Here's how the part is built. I have some questions about the finished solid (model axes, mm). A direction names the side the tool comes from. Coordinates: 2 decimals unless noted, no trailing zeros. Write each loop counter-clockwise with the first axis right and the second up, starting at its lowest first coordinate (ties: lowest second). Pieces come first, ordered by that corner, then holes.
Item 1: I want a section at A-A (y = 8.75). Please give me the cut outline in (x, z).
Item 2: I want a section at B-B (y = 13). Please give me the cut outline in (x, z), and give its area (3 significant figures).
Item 3: I'm going to push flat-ended pins straight in: P1, Ø2, axis at y = 12.5, z = 1.5, coming from the -X side; P2, Ø1, axis at x = 4, y = 5, coming from the -Z side; P3, Ø3, axis at x = -11.5, y = 6, coming from the +Z side. Where does each tip first touch, or does it pass through?
Item 4: Please list where these lines run through material, in increasing order: line 1 (Y direction, x = 16.5, z = 5); line 2 (Y direction, x = 9, z = 14); line 3 (Y direction, x = -8.5, z = 13).
Item 5: For faces 1 (the face through (-12.65, 4.54, -8.06)), 2 (the face through (5.4, 16.5, 16.4)), 3 (the face through (5.4, 5, -16.4)), which set-ups out of +Z, -Z, +X, -X, +Y, -Y let a thin tool reach every point of the face, with its end or its side?
Item 6: If we mould it in two halves opening along X, with no side actions, what happens to faces 4 (the face through (12.4, 1, -6.5)), 5 (the face through (11, 8, -11)), 6 (the face through (11, 0, -9)), 7 (the face through (16.41, 2.23, -8.54))? For each: pulls with the +X half, pulls with the -X half, needs draft (parallel to the pull), parting line crosses it, or undercut.
from build123d import *

# Parameters (mm, degrees)
CHAMFER_1_SIZE = 0.5


with BuildPart() as part:
    # 草图1 → 旋转1 (revolve)
    with BuildSketch(Plane.XY, mode=Mode.PRIVATE) as revolve_1_sk:
        Polygon((14, 0), (14, 2), (15, 2), (15, 7), (16.15, 7), (16.15, 8), (15, 8), (15, 11), (17.65, 11), (17.65, 12), (16.5, 12), (16.5, 16.5), (18.55, 16.5), (19.05, 16), (19.05, 5.5), (18.55, 5), (17, 5), (17, 4), (18.5, 4), (18.5, 0.5), (18, 0), align=None)
    revolve(revolve_1_sk.sketch.rotate(Axis((0, 0, 0), (0, 1, 0)), 90), axis=Axis((0, 0, 0), (0, 1, 0)))  # turned: the seam where the file's is

    # 倒角1
    chamfer_1_edges = [part.edges().sort_by_distance(p)[0] for p in [
        (0, 11, 15),
        (0, 16.5, 16.5),
    ]]
    chamfer(chamfer_1_edges, length=CHAMFER_1_SIZE)


solid = part.part
Answer:
1. outline: circle Ø38.1 at (0, 0); hole circle Ø30 at (0, 0)
2. outline: circle Ø38.1 at (0, 0); hole circle Ø33 at (0, 0)
2. area: 285 mm2
3. P1: stops at x = -19.04
3. P2: stops at z = -18.64
3. P3: stops at z = 16.21
4. line 1: y = 0 to 4, 5 to 11, 12 to 16.5
4. line 2: y = 0 to 11, 12 to 16.14
4. line 3: y = 0 to 7, 8 to 11
5. face 1: +Y
5. face 2: +Z, -Z, +X, -X, +Y
5. face 3: none
6. face 4: undercut
6. face 5: undercut
6. face 6: needs draft
6. face 7: parting line crosses it
